Work out the finished part from the listing and answer in its coordinate system (mm). Face numbers are marked on the shaded views. Coordinates: 2 decimals unless noted, no trailing zeros. Loops run counter-clockwise (first coordinate to the right, second up) from the corner with the lowest first, then second, coordinate; pieces in that order, holes last.
```python
from build123d import *

# Parameters (mm, degrees)
BOSS_EXTRUDE1_DEPTH = 4.572
SKETCH2_W           = 38.1
SKETCH2_H           = 3.2004
CUT_EXTRUDE1_DEPTH  = 5.572
SKETCH3_W           = 38.1
SKETCH3_H           = 6.35
BOSS_EXTRUDE2_DEPTH = 4.572


with BuildPart() as part:
    # Sketch1 → Boss-Extrude1 (new body)
    with BuildSketch(Plane.XY):
        Polygon((-27.0891, 18.738007515), (27.0891, 18.738007515), (30.7594, -21.276818659), (-30.7594, -21.276818659), align=None)
    extrude(amount=BOSS_EXTRUDE1_DEPTH)

    # Sketch2 → Cut-Extrude1 (cut, through all)
    with BuildSketch(Plane.XY.offset(4.572)):
        with Locations((0, 17.137807515)):
            Rectangle(SKETCH2_W, SKETCH2_H)
        Polygon((-30.160830215, -14.751012621), (-27.840792288, 10.542809234), (-23.287904354, 10.125202407), (-25.607942281, -15.168619448), align=None)
        Polygon((27.840792288, 10.542809234), (30.160830215, -14.751012621), (25.607942281, -15.168619448), (23.287904354, 10.125202407), align=None)
    extrude(amount=-CUT_EXTRUDE1_DEPTH, mode=Mode.SUBTRACT)

    # Sketch3 → Boss-Extrude2 (add)
    with BuildSketch(Plane.XY.offset(4.572)):
        with Locations((0, -24.451818659)):
            Rectangle(SKETCH3_W, SKETCH3_H)
    extrude(amount=-BOSS_EXTRUDE2_DEPTH)


solid = part.part
```
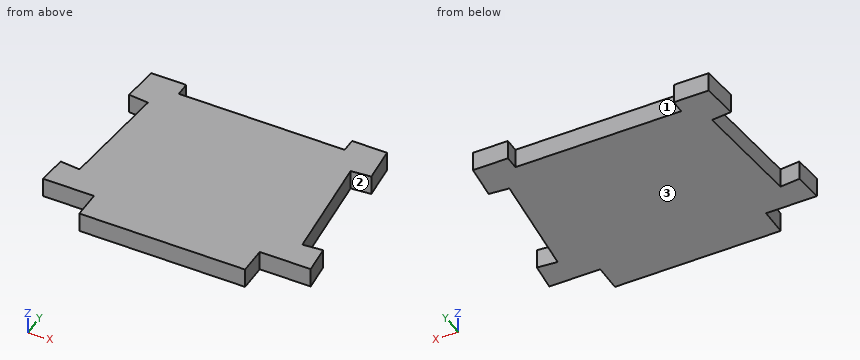
1. Straight lines are drawn through the part: probe 1 along Y at (x, z) = (16, 1.65); probe 2 along Y at (x, z) = (-26.5, 2.65); probe 3 along Y at (x, z) = (-20, 2.4). For each, find the intervals that lie inside material, in ascending order.
2. A cutting plane is placed at A-A, the plane z = 0.85. Give the vertices of the cut face in (x, y).
3. Each of these flat-tipped pins is pushed along its axis until it touches: P1, Ø2, axis at x = -14, z = 2.5, coming from the +Y side; P2, Ø2.5, axis at y = -24, z = 1.5, coming from the -X side; P3, Ø1.4, axis at x = -25, z = 2, coming from the -Y side. Where does it stop, or does it pass through?
4. A cutting plane is placed at B-B, the plane x = 2. Give the vertices of the cut face in (y, z), then the cut area to 3 significant figures.
5. A cutting plane is placed at C-C, the plane y = -23.5. Give the vertices of the cut face in (x, z).
6. Determine the mould class of the marked faces 1, 2 and 3 for opening direction X: released by +X, released by -X, zero draft, split by the parting line, or undercut.
Answers below:
1. probe 1: y = -27.63 to 15.54
1. probe 2: y = -21.28 to -15.09, 10.42 to 18.74
1. probe 3: y = -21.28 to 18.74
2. outline: (-30.76, -21.28) - (-19.05, -21.28) - (-19.05, -27.63) - (19.05, -27.63) - (19.05, -21.28) - (30.76, -21.28) - (30.16, -14.75) - (25.61, -15.17) - (23.29, 10.13) - (27.84, 10.54) - (27.09, 18.74) - (19.05, 18.74) - (19.05, 15.54) - (-19.05, 15.54) - (-19.05, 18.74) - (-27.09, 18.74) - (-27.84, 10.54) - (-23.29, 10.13) - (-25.61, -15.17) - (-30.16, -14.75) - close
3. P1: stops at y = 15.54
3. P2: stops at x = -19.05
3. P3: stops at y = -21.28
4. outline: (-27.63, 0) - (15.54, 0) - (15.54, 4.57) - (-27.63, 4.57) - close
4. area: 197 mm2
5. outline: (-19.05, 0) - (19.05, 0) - (19.05, 4.57) - (-19.05, 4.57) - close
6. face 1: undercut
6. face 2: released by +X
6. face 3: zero draft
